```python
from build123d import *

# Parameters (mm, degrees)
F0_W     = 57.32
F0_H     = 28.2
F1_DEPTH = 19.05
F2_R     = 5
F5_DEPTH = 10.6
F6_R     = 1.25
F7_DEPTH = 1.13


with BuildPart() as f1:
    # F0 (on Top) → F1 (new body)
    with BuildSketch(Plane.XY):
        Rectangle(F0_W, F0_H)
    extrude(amount=F1_DEPTH)

    # F2
    f2_edges = [f1.edges().sort_by_distance(p)[0] for p in [
        (-28.66, 14.1, 9.525),
        (-28.66, -14.1, 9.525),
        (28.66, -14.1, 9.525),
        (28.66, 14.1, 9.525),
    ]]
    fillet(f2_edges, radius=F2_R)

    # F4 (on offset) → F5 (join)
    with BuildSketch(Plane.XY.offset(15.25)):
        with BuildLine():
            Line((-27.716206, 5.95), (-29.45, 5.95))
            ThreePointArc((-29.45, 5.95), (-35.4, 0), (-29.45, -5.95))
            Line((-29.45, -5.95), (-27.716206, -5.95))
            Line((-27.716206, -5.95), (-27.716206, 5.95))
        make_face()
        with BuildLine():
            Line((27.716206, -5.95), (29.45, -5.95))
            ThreePointArc((29.45, -5.95), (35.4, 0), (29.45, 5.95))
            Line((29.45, 5.95), (27.716206, 5.95))
            Line((27.716206, 5.95), (27.716206, -5.95))
        make_face()
    extrude(amount=-F5_DEPTH)

    # F6 (on face) → F7 (join)
    with BuildSketch(Plane.XY.offset(19.05)):
        with Locations((-14.7, 0)):
            Circle(F6_R)
        with Locations((-4.9, 0)):
            Circle(F6_R)
        with Locations((4.9, 0)):
            Circle(F6_R)
        with Locations((14.7, 0)):
            Circle(F6_R)
    extrude(amount=F7_DEPTH)


solid = f1.part
```
Geometry: final body of the model. Coordinates: model frame, mm. A direction names the side the tool comes from. Give positions to 0.01 mm unless a question says otherwise; leave off trailing zeros. Write each loop counter-clockwise with the first axis right and the second up, starting at its lowest first coordinate (ties: lowest second). Pieces come first, ordered by that corner, then holes.
1. Line query: probe 1 along X at (y, z) = (0.5, 19.25); probe 2 along Z at (x, y) = (-23, 6.25); probe 3 along X at (y, z) = (1, 17). Output: solid intervals per line, ascending.
2. Section query B-B, the plane x = 14.7. Return loops of the section in (y, z), then the cut area to 3 significant figures.
3. Reachability of faces 1 (the flat face through (31, 0, 4.65)), 2 (the cylindrical face through (15.855, -0.479, 19.607)), 3 (the flat face through (-31, 0, 4.65)), 4 (the flat face through (31, 0, 15.25)) from +Z, -Z, +X, -X, +Y, -Y: full face, straight path, thin tool, end or side. Return the list, or none.
4. Section query C-C, the plane y = 8.25. Return loops of the section in (x, z), then the cut area to 3 significant figures.
5. Section query D-D, the plane y = 2.25. Return loops of the section in (x, z).
6. Pin query (flat end, axial travel): P1, Ø7.5, axis at x = -33.5, y = -1.5, coming from the -Z side; P2, Ø5, axis at y = -11, z = 14.5, coming from the -X side; P3, Ø3.5, axis at x = 32, y = 2.5, coming from the +Z side. Return the tip coordinate at first contact, or that it passes through.
7. Section query A-A, the plane z = 12.25. Return loops of the section in (x, y).
Computed:
1. probe 1: x = -15.85 to -13.55, -6.05 to -3.75, 3.75 to 6.05, 13.55 to 15.85
1. probe 2: z = 0 to 19.05
1. probe 3: x = -28.66 to 28.66
2. outline: (-14.1, 0) - (14.1, 0) - (14.1, 19.05) - (1.25, 19.05) - (1.25, 20.18) - (-1.25, 20.18) - (-1.25, 19.05) - (-14.1, 19.05) - close
2. area: 540 mm2
3. face 1: -Z, +X, +Y, -Y
3. face 2: +Z
3. face 3: -Z, -X, +Y, -Y
3. face 4: +Z, +X, +Y, -Y
4. outline: (-28.66, 0) - (28.66, 0) - (28.66, 19.05) - (-28.66, 19.05) - close
4. area: 1,090 mm2
5. outline: (-34.96, 4.65) - (-28.66, 4.65) - (-28.66, 0) - (28.66, 0) - (28.66, 4.65) - (34.96, 4.65) - (34.96, 15.25) - (28.66, 15.25) - (28.66, 19.05) - (-28.66, 19.05) - (-28.66, 15.25) - (-34.96, 15.25) - close
6. P1: stops at z = 4.65
6. P2: stops at x = -28.66
6. P3: stops at z = 15.25
7. outline: (-29.45, -5.95) - (-28.66, -5.95) - (-28.66, -9.1) arc R5 ccw to (-23.66, -14.1) - (23.66, -14.1) arc R5 ccw to (28.66, -9.1) - (28.66, -5.95) - (29.45, -5.95) arc R5.95 ccw to (29.45, 5.95) - (28.66, 5.95) - (28.66, 9.1) arc R5 ccw to (23.66, 14.1) - (-23.66, 14.1) arc R5 ccw to (-28.66, 9.1) - (-28.66, 5.95) - (-29.45, 5.95) arc R5.95 ccw to start
